For this review, take the finished solid that the model builds, in its own axes (mm). A direction names the side the tool comes from. Give positions to 0.01 mm unless a question says otherwise; leave off trailing zeros. Order: outer loops, then holes, each group sorted by start corner. A loop starts at its lowest first (then second) coordinate and runs counter-clockwise, first axis right, second up. Notation, with made-up numbers: (39.5, 60.5) - (81.5, 60.5) arc R11 cw to (81.5, 75.5) - close; hole circle Ø5 at (-12.5, 33.5). An arc over 180 degrees is marked (long way). Use a Markdown table: item, result. Add a question column.
1) Wall thickness on L1, parallel to Y at x = -5, z = 13; L2, parallel to X at y = -4.75, z = 5.25; L3, parallel to Z at x = 17.5, y = -1.5: over which ranges is each line inside the solid? List them lowest first.
2) Machinability: for faces 1 (the face through (-44, -5, 8)), 2 (the face through (-1, 0, 11)), which of the approach directions +Z, -Z, +X, -X, +Y, -Y give a long, thin tool a straight path to every point of the face, cutting with its end or side? Answer none if there is none.
3) We need section C-C on x = -5. Write out the cut boundary in (y, z).
4) We need section D-D on z = 14. Write out the cut boundary in (x, y).
5) We need section B-B on z = 3.5. Write out the cut boundary in (x, y), then the cut area to 3 significant figures.
6) Clearance check with flat-ended pins moving along their axes: P1, Ø5, axis at x = 3, y = -8.5, coming from the -Z side; P2, Ø6, axis at x = -39.5, y = -3.5, coming from the -Z side. State where each tip first meets the part, or that it passes through.
7) Mouldability with a two-part tool opening along X and no side actions: class faces 3 (the face through (-1, -10, 11)), 4 (the face through (49.14, -4.93, 14.1)), 5 (the face through (-1, -6, 10)) as released by +X, released by -X, zero draft, split by the parting line, or undercut.
8) We need section A-A on y = -5. Write out the cut boundary in (x, z).
```python
from build123d import *

# Parameters (mm, degrees)
F1_DEPTH = 10
F3_D     = 2


with BuildPart() as f1:
    # F0 (on Front) → F1 (new body)
    with BuildSketch(Plane.XZ):
        with BuildLine():
            ThreePointArc((-50, 2), (-49.414214, 0.585786), (-48, 0))
            Line((-48, 0), (-47, 0))
            ThreePointArc((-47, 0), (-45.585786, 0.585786), (-45, 2))
            Line((-45, 2), (-45, 5))
            ThreePointArc((-45, 5), (-43.535534, 8.535534), (-40, 10))
            Line((-40, 10), (0, 10))
            Line((0, 10), (40, 10))
            ThreePointArc((40, 10), (43.535534, 8.535534), (45, 5))
            Line((45, 5), (45, 2))
            ThreePointArc((45, 2), (45.585786, 0.585786), (47, 0))
            Line((47, 0), (48, 0))
            ThreePointArc((48, 0), (49.414214, 0.585786), (50, 2))
            Line((50, 2), (50, 12))
            ThreePointArc((50, 12), (49.12132, 14.12132), (47, 15))
            Line((47, 15), (0, 15))
            Line((0, 15), (-47, 15))
            ThreePointArc((-47, 15), (-49.12132, 14.12132), (-50, 12))
            Line((-50, 12), (-50, 2))
        make_face()
    extrude(amount=F1_DEPTH)

    # F3 (through all)
    with Locations(Plane.XY.offset(15)):
        with Locations((-5, -5), (5, -5), (0, -5)):
            Hole(F3_D / 2)


solid = f1.part
```
Checked values:
| question | item | result |
|---|---|---|
| 1 | L1 | -10 to -6, -4 to 0 |
| 1 | L2 | -50 to -44.99, 44.99 to 50 |
| 1 | L3 | 10 to 15 |
| 2 | face 1 | -Z, +Y, -Y |
| 2 | face 2 | +Z, -Z, +X, -X, +Y |
| 3 | outline | (-10, 10) - (-6, 10) - (-6, 15) - (-10, 15) - close; (-4, 10) - (0, 10) - (0, 15) - (-4, 15) - close |
| 4 | outline | (-49.24, -10) - (49.24, -10) - (49.24, 0) - (-49.24, 0) - close; hole circle Ø2 at (-5, -5); hole circle Ø2 at (0, -5); hole circle Ø2 at (5, -5) |
| 5 | outline | (-50, -10) - (-45, -10) - (-45, 0) - (-50, 0) - close; (45, -10) - (50, -10) - (50, 0) - (45, 0) - close |
| 5 | area | 100 mm² |
| 6 | P1 | z = 10 |
| 6 | P2 | z = 9.33 |
| 7 | face 3 | zero draft |
| 7 | face 4 | released by +X |
| 7 | face 5 | undercut |
| 8 | outline | (-50, 2) arc R2 ccw to (-48, 0) - (-47, 0) arc R2 ccw to (-45, 2) - (-45, 5) arc R5 cw to (-40, 10) - (-6, 10) - (-6, 15) - (-47, 15) arc R3 ccw to (-50, 12) - close; (-4, 10) - (-1, 10) - (-1, 15) - (-4, 15) - close; (1, 10) - (4, 10) - (4, 15) - (1, 15) - close; (6, 10) - (40, 10) arc R5 cw to (45, 5) - (45, 2) arc R2 ccw to (47, 0) - (48, 0) arc R2 ccw to (50, 2) - (50, 12) arc R3 ccw to (47, 15) - (6, 15) - close |
